```python
from build123d import *

# Parameters (mm, degrees)
SKETCH1_W           = 50
SKETCH1_H           = 50
SKETCH1_R           = 1.1
SKETCH1_W_2         = 10
SKETCH1_H_2         = 3
BOSS_EXTRUDE1_DEPTH = 3
FILLET1_R           = 5


with BuildPart() as part:
    # Sketch1 → Boss-Extrude1 (new body)
    with BuildSketch(Plane(origin=(0, 0, 0), x_dir=(1, 0, 0), z_dir=(0, 1, 0))):
        Rectangle(SKETCH1_W, SKETCH1_H)
        with Locations(Location((-15, 0, 0), (0, 0, 270))):
            Circle(SKETCH1_R, mode=Mode.SUBTRACT)
        with Locations(Location((15, 0, 0), (0, 0, 90))):
            Circle(SKETCH1_R, mode=Mode.SUBTRACT)
        with Locations(Location((-20, 20, 0), (0, 0, 270))):
            Circle(SKETCH1_R, mode=Mode.SUBTRACT)
        with Locations(Location((20, 20, 0), (0, 0, 90))):
            Circle(SKETCH1_R, mode=Mode.SUBTRACT)
        with Locations(Location((20, -20, 0), (0, 0, 270))):
            Circle(SKETCH1_R, mode=Mode.SUBTRACT)
        with Locations(Location((-20, -20, 0), (0, 0, 90))):
            Circle(SKETCH1_R, mode=Mode.SUBTRACT)
        with Locations(Location((0, 15, 0), (0, 0, 270))):
            Circle(SKETCH1_R, mode=Mode.SUBTRACT)
        with Locations(Location((0, -15, 0), (0, 0, 90))):
            Circle(SKETCH1_R, mode=Mode.SUBTRACT)
        Rectangle(SKETCH1_W_2, SKETCH1_H_2, mode=Mode.SUBTRACT)
    extrude(amount=BOSS_EXTRUDE1_DEPTH)

    # Fillet1
    fillet1_edges = [part.edges().sort_by_distance(p)[0] for p in [
        (25, 1.5, 25),
        (-25, 1.5, 25),
        (-25, 1.5, -25),
        (25, 1.5, -25),
    ]]
    fillet(fillet1_edges, radius=FILLET1_R)


solid = part.part
```
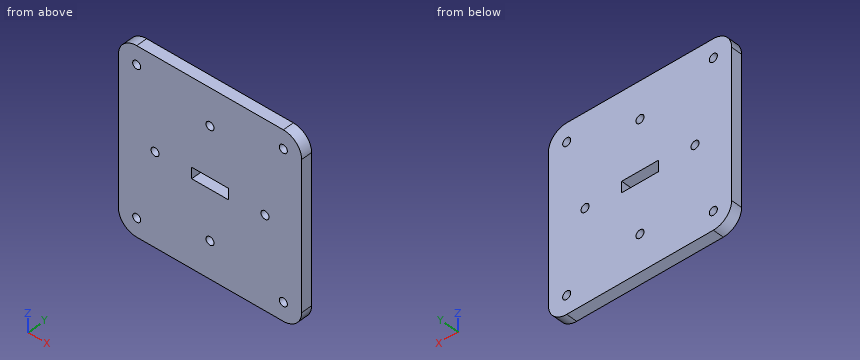
Could you check a few things on this model? Use its own coordinates, in mm. Coordinates: 2 decimals unless noted, no trailing zeros. Loops run counter-clockwise (first coordinate to the right, second up) from the corner with the lowest first, then second, coordinate; pieces in that order, holes last.
1) Will this pin go through, and if not, where does the flat tip stop? pin 1 Ø1.8 at (x, z) = (15, 0) entering from -Y.
Reported:
pin 1: passes through
2) Imagine slicing it at C-C (z = 0). List the corners of the cut face in (x, y) for me.
Reported:
outline: (-25, 0) - (-16.1, 0) - (-16.1, 3) - (-25, 3) - close; (-13.9, 0) - (-5, 0) - (-5, 3) - (-13.9, 3) - close; (5, 0) - (13.9, 0) - (13.9, 3) - (5, 3) - close; (16.1, 0) - (25, 0) - (25, 3) - (16.1, 3) - close
3) Please list where these lines run through material, in increasing order: line 1 along X through (y, z) = (1.95, 20); line 2 along Z through (x, y) = (-1, 1.45); line 3 along X through (y, z) = (1.8, 0).
Reported:
line 1: x = -25 to -21.1, -18.9 to 18.9, 21.1 to 25
line 2: z = -25 to -15.46, -14.54 to -1.5, 1.5 to 14.54, 15.46 to 25
line 3: x = -25 to -16.1, -13.9 to -5, 5 to 13.9, 16.1 to 25
4) Imagine slicing it at D-D (y = 1.7). State how many separate pieces and enclosed holes the cut face has, and give its area (3 significant figures).
Reported:
separate pieces: 1
enclosed holes: 9
area: 2,420 mm2
5) Imagine slicing it at B-B (x = 0). List the corners of the cut face in (y, z) for me, and give its area (3 significant figures).
Reported:
outline: (0, -25) - (3, -25) - (3, -16.1) - (0, -16.1) - close; (0, -13.9) - (3, -13.9) - (3, -1.5) - (0, -1.5) - close; (0, 1.5) - (3, 1.5) - (3, 13.9) - (0, 13.9) - close; (0, 16.1) - (3, 16.1) - (3, 25) - (0, 25) - close
area: 128 mm2
6) Imagine slicing it at A-A (x = -15). List the corners of the cut face in (y, z) for me, and give its area (3 significant figures).
Reported:
outline: (0, -25) - (3, -25) - (3, -1.1) - (0, -1.1) - close; (0, 1.1) - (3, 1.1) - (3, 25) - (0, 25) - close
area: 143 mm2
